The listing builds one solid part. Answer for the finished solid, in the listing's coordinates (mm). Give positions to 0.01 mm unless a question says otherwise; leave off trailing zeros. Write each loop counter-clockwise with the first axis right and the second up, starting at its lowest first coordinate (ties: lowest second). Pieces come first, ordered by that corner, then holes. Notation, with made-up numbers: M 11,-6 L 58,-6 A22 ccw 58,32 Z; hole C -12.75,-32.5 d7. An arc over 180 degrees is marked long. Answer as a JSON object with one key per item and string values.
```python
from build123d import *

# Parameters (mm, degrees)
ESBO_O1_W                    = 205
ESBO_O1_H                    = 268
RESSALTO_EXTRUS_O1_DEPTH     = 6
ESBO_O3_R                    = 23.9
ESBO_O3_R_2                  = 2.1
CORTE_EXTRUS_O4_DEPTH        = 169.814247029
ESBO_O4_R                    = 15
CORTE_EXTRUS_O5_DEPTH        = 169.814247029
FURO_DE_DI_METRO_4_2_4_2_1_D = 4.2


with BuildPart() as part:
    # Esboço1 → Ressalto-extrusão1 (new body)
    with BuildSketch(Plane.XZ):
        Rectangle(ESBO_O1_W, ESBO_O1_H)
    extrude(amount=-RESSALTO_EXTRUS_O1_DEPTH)

    # Esboço3 → Corte-extrusão4 (cut, through all)
    with BuildSketch(Plane(origin=(0, 6, 0), x_dir=(1, 0, 0), z_dir=(0, 1, 0))):
        with Locations(Location((-52.5, 1, 0), (0, 0, 270))):
            Circle(ESBO_O3_R)
        with Locations(Location((-72.5, 21, 0), (0, 0, 270))):
            Circle(ESBO_O3_R_2)
        with Locations(Location((-32.5, 21, 0), (0, 0, 270))):
            Circle(ESBO_O3_R_2)
        with Locations(Location((-32.5, -19, 0), (0, 0, 270))):
            Circle(ESBO_O3_R_2)
        with Locations(Location((-72.5, -19, 0), (0, 0, 270))):
            Circle(ESBO_O3_R_2)
    extrude(amount=-CORTE_EXTRUS_O4_DEPTH, mode=Mode.SUBTRACT)

    # Esboço4 → Corte-extrusão5 (cut, through all)
    with BuildSketch(Plane(origin=(0, 6, 0), x_dir=(1, 0, 0), z_dir=(0, 1, 0))):
        with Locations(Location((50, 30, 0), (0, 0, 270))):
            Circle(ESBO_O4_R)
        with Locations(Location((50, -30, 0), (0, 0, 270))):
            Circle(ESBO_O4_R)
        with Locations(Location((50, 90, 0), (0, 0, 270))):
            Circle(ESBO_O4_R)
        with Locations(Location((50, -90, 0), (0, 0, 270))):
            Circle(ESBO_O4_R)
    extrude(amount=-CORTE_EXTRUS_O5_DEPTH, mode=Mode.SUBTRACT)

    # Furo de diâmetro Ø4.2 (4.2)1 (through all)
    with Locations(Plane(origin=(0, 6, 0), x_dir=(1, 0, 0), z_dir=(0, 1, 0))):
        with Locations((-87.5, 116), (-18, 116), (28.5, 116), (78, 116), (-77.5, -117), (-28, -117), (18.5, -117), (88, -117)):
            Hole(FURO_DE_DI_METRO_4_2_4_2_1_D / 2)


solid = part.part
```
1. A cutting plane is placed at B-B, the plane y = 3.4. Count the separate pieces of the cut face and the enclosed holes in it, plus the area to 3 significant figures.
Verdict:
{"separate pieces": "1", "enclosed holes": "17", "area": "50,200 mm2"}
2. Consider line 1 along X through (y, z) = (2.8, 117); line 2 along X through (y, z) = (4.05, -90); line 3 along Z through (x, y) = (-87.5, 4). Determine where each line is inside the solid, lowest interval first.
Verdict:
{"line 1": "x = -102.5 to -79.6, -75.4 to -30.1, -25.9 to 16.4, 20.6 to 85.9, 90.1 to 102.5", "line 2": "x = -102.5 to 35, 65 to 102.5", "line 3": "z = -134 to -118.1, -113.9 to 134"}
3. A cutting plane is placed at A-A, the plane z = 99. Give the vertices of the cut face in (x, y), plus the area to 3 significant figures.
Verdict:
{"outline": "M -102.5,0 L 38,0 L 38,6 L -102.5,6 Z; M 62,0 L 102.5,0 L 102.5,6 L 62,6 Z", "area": "1,090 mm2"}
4. A cutting plane is placed at C-C, the plane x = 47. Give the vertices of the cut face in (y, z).
Verdict:
{"outline": "M 0,-134 L 6,-134 L 6,-104.7 L 0,-104.7 Z; M 0,-75.3 L 6,-75.3 L 6,-44.7 L 0,-44.7 Z; M 0,-15.3 L 6,-15.3 L 6,15.3 L 0,15.3 Z; M 0,44.7 L 6,44.7 L 6,75.3 L 0,75.3 Z; M 0,104.7 L 6,104.7 L 6,134 L 0,134 Z"}
5. The mould has two halves that part along Z. Classify faces 1 (the flat face through (-102.5, 3, -2)), 2 (the cylindrical face through (60.138, 3.042, -41.056)), 3 (the flat face through (-1, 3, 134)), 4 (the cylindrical face through (-28.8, 3, -4.1)): released by +Z, released by -Z, zero draft, split by the parting line, or undercut.
Verdict:
{"face 1": "zero draft", "face 2": "undercut", "face 3": "released by +Z", "face 4": "undercut"}
6. A cutting plane is placed at D-D, the plane z = 30. Give the vertices of the cut face in (x, y).
Verdict:
{"outline": "M -102.5,0 L 35,0 L 35,6 L -102.5,6 Z; M 65,0 L 102.5,0 L 102.5,6 L 65,6 Z"}
